Answer from the drawing. Dimensions are ordinates in mm from the lowest x, y and z of the part. A direction names the side the tool comes from. Round coordinates to 2 decimals unless told otherwise and drop trailing zeros. Write each loop counter-clockwise with the first axis right and the second up, starting at its lowest first coordinate (ties: lowest second). Pieces come first, ordered by that corner, then holes. Notation, with made-up numbers: (-1.5, 11.25) - (21.5, 11.25) arc R19 ccw to (21.5, 47.25) - close; hole circle Ø9 at (-12.5, -38). An arc over 180 degrees is marked (long way). Answer in a Markdown table with one row per item.
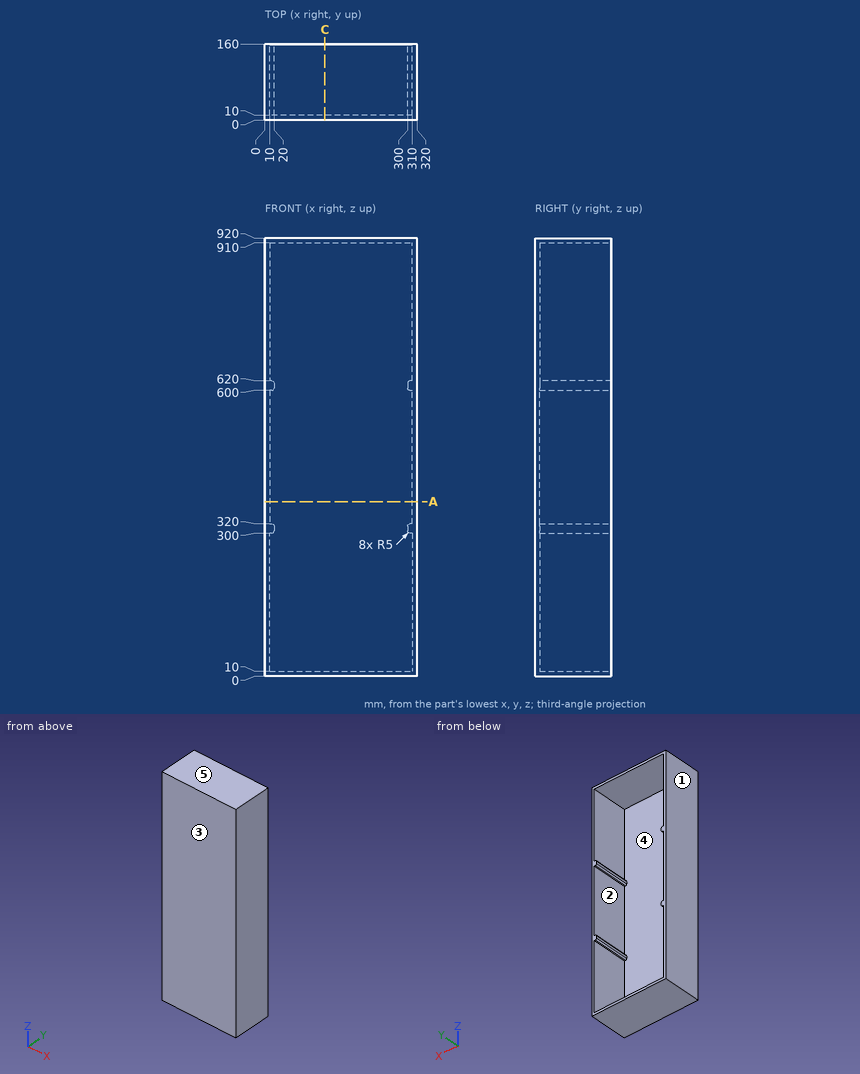
(1) A flat-ended cylindrical pin translates along its axis: pin 1 (3 mm diameter, centred on x = 254.5, z = 180, fed in from -Y). Find the tip coordinate at first contact, or state that the pin passes through.
Checked values:
| item | result |
|---|---|
| pin 1 | stops at y = 0 |
(2) Section A-A (z = 366.5) is taken. Give the vertices of the cut face in (x, y).
Checked values:
| item | result |
|---|---|
| outline | (0, 0) - (320, 0) - (320, 160) - (310, 160) - (310, 10) - (10, 10) - (10, 160) - (0, 160) - close |
(3) For a pull along Z with two mould halves and no side action, classify the marked faces 3, 4 and 5 as pulls with the +Z half, pulls with the -Z half, needs draft (parallel to the pull), parting line crosses it, or undercut.
Checked values:
| item | result |
|---|---|
| face 3 | needs draft |
| face 4 | undercut |
| face 5 | pulls with the +Z half |
(4) For the marked faces 1 and 2, determine the directions among +Z, -Z, +X, -X, +Y, -Y from which every point of the face is accessible in a straight line to the end or side of a thin tool.
Checked values:
| item | result |
|---|---|
| face 1 | +Z, -Z, -X, +Y, -Y |
| face 2 | +Y |
(5) Find the intervals of material crossed by line 1 (X direction, y = 70, z = 291.5); line 2 (Z direction, x = 225, y = 34); line 3 (Y direction, x = 95, z = 49), in increasing order.
Checked values:
| item | result |
|---|---|
| line 1 | x = 0 to 10, 310 to 320 |
| line 2 | z = 0 to 10, 910 to 920 |
| line 3 | y = 0 to 10 |
(6) Section C-C (x = 126.5) is taken. Give the vertices of the cut face in (y, z), and give its area (3 significant figures).
Checked values:
| item | result |
|---|---|
| outline | (0, 0) - (160, 0) - (160, 10) - (10, 10) - (10, 910) - (160, 910) - (160, 920) - (0, 920) - close |
| area | 12,200 mm2 |
